Read the model definition and answer for the solid it produces. Units are mm, in the model's axes. Face numbers are marked on the shaded views. A direction names the side the tool comes from. Round coordinates to 2 decimals unless told otherwise and drop trailing zeros. Order: outer loops, then holes, each group sorted by start corner. A loop starts at its lowest first (then second) coordinate and runs counter-clockwise, first axis right, second up. Notation, with made-up numbers: (-29, 43) -> (-14, 43) arc R29 ccw to (-14, 70) -> close; hole circle Ø5 at (-23.5, 3). An arc over 180 degrees is marked (long way). Use a Markdown table: item, result. Add a question column.
1. The mould has two halves that part along Y. Classify the marked faces 3, 4, 5 and 6: +Y half, -Y half, draft (parallel to the pull), parting line (faces both ways), or undercut.
2. Section D-D, the plane x = -19 is taken. Give the vertices of the cut face in (y, z).
3. Section B-B, the plane y = 41 is taken. Give the vertices of the cut face in (x, z), then the cut area to 3 significant figures.
4. Consider L1, parallel to Y at x = 40, z = 6; L2, parallel to Y at x = -38, z = 2.3; L3, parallel to Y at x = 14, z = 6. Determine where each line is inside the solid, lowest interval first. Write a range as [from, to].
5. Section A-A, the plane x = 0 is taken. Give the vertices of the cut face in (y, z), then the cut area to 3 significant figures.
6. Given pin 1 (3 mm diameter, centred on x = -38, y = -65.5, fed in from +Z); pin 2 (6 mm diameter, centred on x = 0.5, y = -44.5, fed in from +Z); pin 3 (0.8 mm diameter, centred on x = 46.5, z = 12, fed in from -Y); pin 4 (4 mm diameter, centred on x = -39, y = 47.5, fed in from +Z), each flat-ended and moving along its own axis, determine where each tip first touches the part or whether it passes through.
7. For the marked faces 1 and 2, determine the directions among +Z, -Z, +X, -X, +Y, -Y from which every point of the face is accessible in a straight line to the end or side of a thin tool.
8. Section C-C, the plane z = 6 is taken. Give the number of separate pieces and of enclosed holes in the cut face, then the cut area to 3 significant figures.
```python
from build123d import *

# Parameters (mm, degrees)
F0_W      = 96
F0_H      = 152
F1_DEPTH  = 3
F2_W      = 96
F2_H      = 152
F2_W_2    = 91
F2_H_2    = 146
F3_DEPTH  = 15
F4_R      = 1.75
F5_DEPTH  = 3
F6_R      = 5
F7_R      = 5
F8_DEPTH  = 152.001
F9_W      = 11
F9_H      = 8
F10_DEPTH = 5
F11_R     = 1.75
F12_DEPTH = 15.001
F13_DEPTH = 25
F14_R     = 2.5
F15_DEPTH = 3.001
F16_W     = 12
F16_H     = 20.9038736373
F17_DEPTH = 2.501
F18_SIZE  = 0.5
F19_R     = 4.5
F20_DEPTH = 1


with BuildPart() as f1:
    # F0 (on Top) → F1 (new body)
    with BuildSketch(Plane.XY):
        Rectangle(F0_W, F0_H)
    extrude(amount=F1_DEPTH)

    # F2 (on face) → F3 (join)
    with BuildSketch(Plane.XY.offset(3)):
        Rectangle(F2_W, F2_H)
        Rectangle(F2_W_2, F2_H_2, mode=Mode.SUBTRACT)
    extrude(amount=F3_DEPTH)

    # F4 (on face) → F5 (cut, through all)
    with BuildSketch(Plane.XY.offset(3)):
        with Locations((-38, 65.5)):
            Circle(F4_R)
        with Locations((38, 65.5)):
            Circle(F4_R)
        with Locations((-38, -65.5)):
            Circle(F4_R)
        with Locations((38, -65.5)):
            Circle(F4_R)
    extrude(amount=-F5_DEPTH, mode=Mode.SUBTRACT)

    # F6
    f6_edges = [f1.edges().sort_by_distance(p)[0] for p in [
        (-48, -76, 9),
        (48, -76, 9),
        (45.5, -73, 10.5),
        (-45.5, -73, 10.5),
        (-48, 76, 9),
        (-45.5, 73, 10.5),
        (48, 76, 9),
        (45.5, 73, 10.5),
    ]]
    fillet(f6_edges, radius=F6_R)

    # F7 (on face) → F8 (cut, through all)
    with BuildSketch(Plane.XZ.offset(76)):
        with Locations((-28, 18)):
            Circle(F7_R)
        with Locations((0, 18)):
            Circle(F7_R)
        with Locations((28, 18)):
            Circle(F7_R)
    extrude(amount=-F8_DEPTH, mode=Mode.SUBTRACT)

    # F9 (on face) → F10 (join)
    with BuildSketch(Plane.XY.offset(3)):
        with Locations((-40, -53)):
            Rectangle(F9_W, F9_H)
        with Locations((40, -53)):
            Rectangle(F9_W, F9_H)
        with Locations((-40, 47)):
            Rectangle(F9_W, F9_H)
        with Locations((40, 47)):
            Rectangle(F9_W, F9_H)
    extrude(amount=F10_DEPTH)

    # F11 (on face) → F12 (cut, through all)
    with BuildSketch(Plane.XY.offset(3)):
        with Locations((-40, -53)):
            Circle(F11_R)
        with Locations((40, -53)):
            Circle(F11_R)
        with Locations((-40, 47)):
            Circle(F11_R)
        with Locations((40, 47)):
            Circle(F11_R)
    extrude(amount=F12_DEPTH, mode=Mode.SUBTRACT)

    # F11 (on face) → F13 (cut)
    with BuildSketch(Plane.XY.offset(3)):
        with Locations((-40, -53)):
            Circle(F11_R)
        with Locations((40, -53)):
            Circle(F11_R)
        with Locations((-40, 47)):
            Circle(F11_R)
        with Locations((40, 47)):
            Circle(F11_R)
    extrude(amount=-F13_DEPTH, mode=Mode.SUBTRACT)

    # F14 (on face) → F15 (cut, through all)
    with BuildSketch(Plane.XY.offset(3)):
        with Locations((-10, -63)):
            Circle(F14_R)
        with Locations((10, -63)):
            Circle(F14_R)
        with Locations((-10, 63)):
            Circle(F14_R)
        with Locations((10, 63)):
            Circle(F14_R)
    extrude(amount=-F15_DEPTH, mode=Mode.SUBTRACT)

    # F16 (on face) → F17 (cut, through all)
    with BuildSketch(Plane(origin=(45.5, 0, 0), x_dir=(0, -1, 0), z_dir=(-1, 0, 0))):
        with Locations((37, 18.4519368187)):
            Rectangle(F16_W, F16_H)
    extrude(amount=-F17_DEPTH, mode=Mode.SUBTRACT)

    # F18 (call 1 of 7: OpenCascade refuses the feature's edges together)
    f18_edges = [f1.edges().sort_by_distance(p)[0] for p in [
        (48, 20, 18),
    ]]
    chamfer(f18_edges, length=F18_SIZE)

    # F18#2 (call 2 of 7)
    f18_2_edges = [f1.edges().sort_by_distance(p)[0] for p in [
        (48, -57, 18),
        (46.535534, -74.535534, 18),
    ]]
    chamfer(f18_2_edges, length=F18_SIZE)

    # F18#3 (call 3 of 7)
    f18_3_edges = [f1.edges().sort_by_distance(p)[0] for p in [
        (14, -76, 18),
    ]]
    chamfer(f18_3_edges, length=F18_SIZE)

    # F18#4 (call 4 of 7)
    f18_4_edges = [f1.edges().sort_by_distance(p)[0] for p in [
        (-14, -76, 18),
    ]]
    chamfer(f18_4_edges, length=F18_SIZE)

    # F18#5 (call 5 of 7)
    f18_5_edges = [f1.edges().sort_by_distance(p)[0] for p in [
        (-38, -76, 18),
    ]]
    chamfer(f18_5_edges, length=F18_SIZE)

    # F18#6 (call 6 of 7)
    f18_6_edges = [f1.edges().sort_by_distance(p)[0] for p in [
        (-14, 76, 18),
    ]]
    chamfer(f18_6_edges, length=F18_SIZE)

    # F18#7 (call 7 of 7)
    f18_7_edges = [f1.edges().sort_by_distance(p)[0] for p in [
        (14, 76, 18),
    ]]
    chamfer(f18_7_edges, length=F18_SIZE)

    # F19 (on face) → F20 (cut)
    with BuildSketch(Plane.XY.offset(3)):
        with Locations((10, 63)):
            Circle(F19_R)
        with Locations((-10, 63)):
            Circle(F19_R)
        with Locations((10, -63)):
            Circle(F19_R)
        with Locations((-10, -63)):
            Circle(F19_R)
    extrude(amount=-F20_DEPTH, mode=Mode.SUBTRACT)


solid = f1.part
```
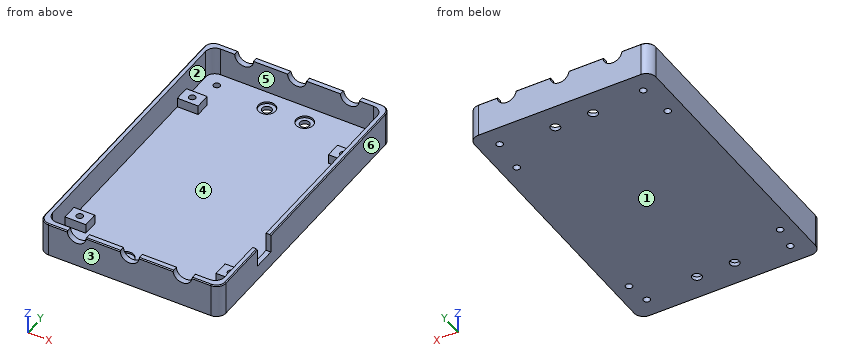
Verdict:
| question | item | result |
|---|---|---|
| 1 | face 3 | -Y half |
| 1 | face 4 | undercut |
| 1 | face 5 | undercut |
| 1 | face 6 | draft |
| 2 | outline | (-76, 0) -> (76, 0) -> (76, 17.5) -> (75.5, 18) -> (73, 18) -> (73, 3) -> (-73, 3) -> (-73, 18) -> (-75.5, 18) -> (-76, 17.5) -> close |
| 3 | outline | (-48, 0) -> (48, 0) -> (48, 17.5) -> (47.5, 18) -> (45.5, 18) -> (45.5, 3) -> (-45.5, 3) -> (-45.5, 18) -> (-47.5, 18) -> (-48, 17.5) -> close |
| 3 | area | 363 mm2 |
| 4 | L1 | y = [-76, -73], [-57, -54.75], [-51.25, -49], [43, 45.25], [48.75, 51], [73, 76] |
| 4 | L2 | y = [-76, -67.25], [-63.75, 63.75], [67.25, 76] |
| 4 | L3 | y = [-76, -73], [73, 76] |
| 5 | outline | (-76, 0) -> (76, 0) -> (76, 13) -> (73, 13) -> (73, 3) -> (-73, 3) -> (-73, 13) -> (-76, 13) -> close |
| 5 | area | 516 mm2 |
| 6 | pin 1 | passes through |
| 6 | pin 2 | stops at z = 3 |
| 6 | pin 3 | stops at y = -74.92 |
| 6 | pin 4 | stops at z = 8 |
| 7 | face 1 | -Z, +X, -X, +Y, -Y |
| 7 | face 2 | +Z |
| 8 | separate pieces | 1 |
| 8 | enclosed holes | 5 |
| 8 | area | 1,620 mm2 |
